Job drawing, mm, ordinate dimensions from the low corner. One solid piece. A direction names the side the tool comes from. Round coordinates to 2 decimals unless told otherwise and drop trailing zeros. Loops run counter-clockwise (first coordinate to the right, second up) from the corner with the lowest first, then second, coordinate; pieces in that order, holes last. Notation, with made-up numbers: M -10.75,12 L 21.25,12 A34 cw 21.25,47 Z; hole C -20.75,43 d1. An arc over 180 degrees is marked long. One line per item, written item: value.
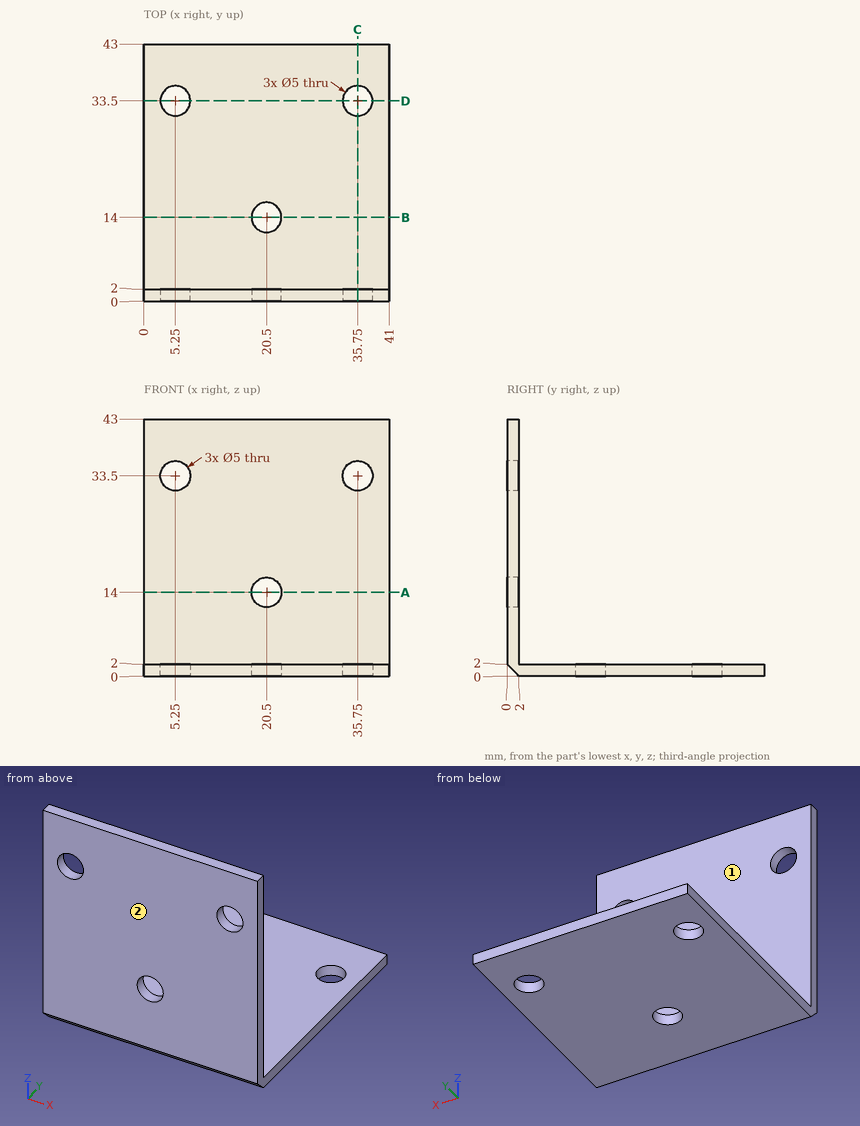
Item 1: Slice it at D-D, the plane y = 33.5. Give the cut face in (x, z).
Check values:
outline: M 0,0 L 2.75,0 L 2.75,2 L 0,2 Z; M 7.75,0 L 33.25,0 L 33.25,2 L 7.75,2 Z; M 38.25,0 L 41,0 L 41,2 L 38.25,2 Z
Item 2: Which spindle directions (+Z, -Z, +X, -X, +Y, -Y) get a long thin tool onto all of the face, cutting with end or side? Do the marked faces 1 and 2. Say none if no direction does.
Check values:
face 1: +Z, +X, -X, +Y
face 2: +Z, -Z, +X, -X, -Y
Item 3: Slice it at C-C, the plane x = 35.75. Give the cut face in (y, z), and give its area (3 significant figures).
Check values:
outline: M 0,2 L 2,0 L 31,0 L 31,2 L 2,2 L 2,31 L 0,31 Z; M 0,36 L 2,36 L 2,43 L 0,43 Z; M 36,0 L 43,0 L 43,2 L 36,2 Z
area: 146 mm2
Item 4: Slice it at A-A, the plane z = 14. Give the cut face in (x, y).
Check values:
outline: M 0,0 L 18,0 L 18,2 L 0,2 Z; M 23,0 L 41,0 L 41,2 L 23,2 Z
Item 5: Drop flat-ended pins along their axis: P1, Ø4, axis at x = 35.75, y = 33.5, coming from the +Z side; P2, Ø6.5, axis at x = 20.5, z = 14, coming from the +Y side; P3, Ø12.5, axis at x = 29, y = 23.5, coming from the +Z side. Give the stop position or say it passes through.
Check values:
P1: passes through
P2: stops at y = 2
P3: stops at z = 2
Item 6: Wall check: line 1 along Y through (x, z) = (35, 24.5); line 2 along Y through (x, z) = (35.75, 0.8). Give the ranges that are in metal, low to high.
Check values:
line 1: y = 0 to 2
line 2: y = 1.2 to 31, 36 to 43
